The model under review builds one solid part; all positions refer to its coordinate system, in mm. Face numbers are marked on the shaded views. A direction names the side the tool comes from. Coordinates: 2 decimals unless noted, no trailing zeros. Order: outer loops, then holes, each group sorted by start corner. A loop starts at its lowest first (then second) coordinate and runs counter-clockwise, first axis right, second up. Notation, with made-up numbers: M 82,-24.5 L 93,-24.5 A25 ccw 93,12.5 Z; hole C 57,69.5 d10. An arc over 180 degrees is marked long. Answer as CSV lines item,"result". Start each with the question number.
Q1. Consider section B-B on x = 8. Write out the cut boundary in (y, z).
Q2. Wall thickness on L1, parallel to Z at x = 1, y = 4.5 (3 decimals); L2, parallel to X at y = 4.25, z = 2.25; L3, parallel to Z at x = -7, y = 4.75: over which ranges is each line inside the solid? List them lowest first. Write a range as [from, to].
Q3. Consider section C-C on y = 5.5. State how many separate pieces and enclosed holes the cut face has, and give its area (3 significant figures).
Q4. For P1, Ø2, axis at x = 2, z = 0.5, coming from the -Y side; P2, Ø0.6, axis at x = 1, y = -2, coming from the +Z side (3 decimals); P3, Ø0.6, axis at y = -1, z = -1, coming from the +X side (3 decimals); P4, Ø4, axis at x = 0, z = 1.5, coming from the +Y side, all flat-tipped, find the tip position at first contact; note any pin that passes through.
Q5. The part is to be moulded in two halves that separate along Z. For the marked faces 3, 4, 5 and 6, say which applies: +Z half, -Z half, draft (parallel to the pull), parting line (faces both ways), or undercut.
Q6. Machinability: for the marked faces 1 and 2, which of the approach directions +Z, -Z, +X, -X, +Y, -Y give a long, thin tool a straight path to every point of the face, cutting with its end or side? Answer none if there is none.
Q7. Consider section A-A on z = 3.75. Write out the cut boundary in (x, y), and give its area (3 significant figures).
from build123d import *

# Parameters (mm, degrees)
SKETCH_1_W           = 25.26
SKETCH_1_H           = 9
EXTRUDE_1_DEPTH      = 9
SKETCH_2_W           = 22.86
SKETCH_2_H           = 6.6
CUT_EXTRUDE_1_DEPTH  = 6.5
SKETCH_3_W           = 4.2
SKETCH_3_H           = 6.5
CUT_EXTRUDE_2_DEPTH  = 6.5
EXTRUDE_2_DEPTH      = 3.5
EXTRUDE_2_DEPTH_BACK = 8
SKETCH_5_W           = 0.75
SKETCH_5_H           = 0.75


with BuildPart() as part:
    # 草图1 → 拉伸1 (new body)
    with BuildSketch(Plane(origin=(0, 0, 0), x_dir=(1, 0, 0), z_dir=(0, 1, 0))):
        Rectangle(SKETCH_1_W, SKETCH_1_H)
    extrude(amount=EXTRUDE_1_DEPTH)

    # 草图2 → 切除-拉伸1 (cut)
    with BuildSketch(Plane(origin=(0, 9, 0), x_dir=(-1, 0, 0), z_dir=(0, 1, 0))):
        Rectangle(SKETCH_2_W, SKETCH_2_H)
    extrude(amount=-CUT_EXTRUDE_1_DEPTH, mode=Mode.SUBTRACT)

    # 草图3 → 切除-拉伸2 (cut)
    with BuildSketch(Plane.XY.offset(4.5)):
        with Locations((0, 5.75)):
            Rectangle(SKETCH_3_W, SKETCH_3_H)
    extrude(amount=-CUT_EXTRUDE_2_DEPTH, mode=Mode.SUBTRACT)

    # 草图5 → 拉伸2 (add, two sides: drawn at the far end of the back side and taken through both)
    with BuildSketch(Plane.XZ.offset(-EXTRUDE_2_DEPTH_BACK)):
        with Locations((-1.27, 1.27)):
            Rectangle(SKETCH_5_W, SKETCH_5_H)
        with Locations((-3.81, 1.27)):
            Rectangle(SKETCH_5_W, SKETCH_5_H)
        with Locations((-6.35, 1.27)):
            Rectangle(SKETCH_5_W, SKETCH_5_H)
        with Locations((-8.89, 1.27)):
            Rectangle(SKETCH_5_W, SKETCH_5_H)
        with Locations((-8.89, -1.27)):
            Rectangle(SKETCH_5_W, SKETCH_5_H)
        with Locations((-6.35, -1.27)):
            Rectangle(SKETCH_5_W, SKETCH_5_H)
        with Locations((-3.81, -1.27)):
            Rectangle(SKETCH_5_W, SKETCH_5_H)
        with Locations((-1.27, -1.27)):
            Rectangle(SKETCH_5_W, SKETCH_5_H)
        with Locations((1.27, -1.27)):
            Rectangle(SKETCH_5_W, SKETCH_5_H)
        with Locations((3.81, -1.27)):
            Rectangle(SKETCH_5_W, SKETCH_5_H)
        with Locations((6.35, -1.27)):
            Rectangle(SKETCH_5_W, SKETCH_5_H)
        with Locations((8.89, -1.27)):
            Rectangle(SKETCH_5_W, SKETCH_5_H)
        with Locations((8.89, 1.27)):
            Rectangle(SKETCH_5_W, SKETCH_5_H)
        with Locations((6.35, 1.27)):
            Rectangle(SKETCH_5_W, SKETCH_5_H)
        with Locations((3.81, 1.27)):
            Rectangle(SKETCH_5_W, SKETCH_5_H)
        with Locations((1.27, 1.27)):
            Rectangle(SKETCH_5_W, SKETCH_5_H)
    extrude(amount=EXTRUDE_2_DEPTH + EXTRUDE_2_DEPTH_BACK)


solid = part.part
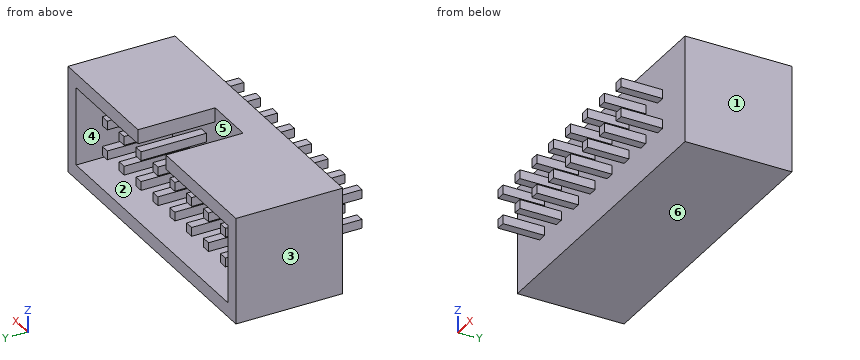
Evaluation:
1,outline,"M 0,-4.5 L 9,-4.5 L 9,-3.3 L 2.5,-3.3 L 2.5,3.3 L 9,3.3 L 9,4.5 L 0,4.5 Z"
2,L1,"z = [-4.5, -3.3], [-1.645, -0.895], [0.895, 1.645]"
2,L2,"x = [-12.63, -11.43], [11.43, 12.63]"
2,L3,"z = [-4.5, -3.3], [3.3, 4.5]"
3,separate pieces,"17"
3,enclosed holes,"0"
3,area,"80.4 mm²"
4,P1,"stops at y = -3.5"
4,P2,"stops at z = 1.645"
4,P3,"stops at x = 9.265"
4,P4,"stops at y = 8"
5,face 3,"draft"
5,face 4,"undercut"
5,face 5,"undercut"
5,face 6,"-Z half"
6,face 1,"+Z, -Z, +X, +Y, -Y"
6,face 2,"+Y"
7,outline,"M -12.63,0 L 12.63,0 L 12.63,9 L 2.1,9 L 2.1,2.5 L -2.1,2.5 L -2.1,9 L -12.63,9 Z"
7,area,"200 mm²"
